from build123d import *

# Parameters (mm, degrees)
SKETCH1_W            = 28
SKETCH1_H            = 22
BOSS_EXTRUDE1_DEPTH  = 32
SKETCH21_W           = 26
SKETCH21_H           = 23
CUT_EXTRUDE10_DEPTH  = 17
SKETCH22_W           = 4
SKETCH22_H           = 8.5
CUT_EXTRUDE11_DEPTH  = 35.885527085
SKETCH23_W           = 10
SKETCH23_H           = 5
CUT_EXTRUDE12_DEPTH  = 5
SKETCH24_W           = 26
SKETCH24_H           = 24
BOSS_EXTRUDE4_DEPTH  = 15
BOSS_EXTRUDE5_DEPTH  = 28
SKETCH26_W           = 28
SKETCH26_H           = 21
SKETCH26_W_2         = 10
SKETCH26_H_2         = 5
BOSS_EXTRUDE6_DEPTH  = 2
BOSS_EXTRUDE7_DEPTH  = 2
FILLET1_R            = 5
FILLET2_R            = 10
SKETCH31_W           = 2
SKETCH31_H           = 26
BOSS_EXTRUDE8_DEPTH  = 0.5
BOSS_EXTRUDE12_DEPTH = 1
SKETCH41_W           = 2
SKETCH41_H           = 4
BOSS_EXTRUDE15_DEPTH = 3.5
SKETCH44_W           = 7
SKETCH44_H           = 6
BOSS_EXTRUDE17_DEPTH = 1
SKETCH30_R           = 1.25
CUT_EXTRUDE13_DEPTH  = 6
BOSS_EXTRUDE9_DEPTH  = 4
SKETCH37_W           = 1
SKETCH37_H           = 27
BOSS_EXTRUDE13_DEPTH = 0.5
SKETCH38_W           = 3
SKETCH38_H           = 2.5
CUT_EXTRUDE15_DEPTH  = 8
CUT_EXTRUDE16_DEPTH  = 6
SKETCH45_W           = 3
SKETCH45_H           = 6
CUT_EXTRUDE18_DEPTH  = 7
BOSS_EXTRUDE18_START = 1
BOSS_EXTRUDE18_DEPTH = 1
SKETCH48_W           = 10
SKETCH48_H           = 5
CUT_EXTRUDE19_DEPTH  = 60.958318856


with BuildPart() as part:
    # Sketch1 → Boss-Extrude1 (new body)
    with BuildSketch(Plane(origin=(0, 0, 0), x_dir=(1, 0, 0), z_dir=(0, 1, 0))):
        Rectangle(SKETCH1_W, SKETCH1_H)
    extrude(amount=BOSS_EXTRUDE1_DEPTH)

    # Sketch21 → Cut-Extrude10 (cut)
    with BuildSketch(Plane.XY.offset(11)):
        with Locations((1, 13.5)):
            Rectangle(SKETCH21_W, SKETCH21_H)
    extrude(amount=-CUT_EXTRUDE10_DEPTH, mode=Mode.SUBTRACT)

    # Sketch22 → Cut-Extrude11 (cut, through all)
    with BuildSketch(Plane(origin=(0, 2, 0), x_dir=(1, 0, 0), z_dir=(0, 1, 0))):
        with Locations((-6, 0)):
            Rectangle(SKETCH22_W, SKETCH22_H)
    extrude(amount=-CUT_EXTRUDE11_DEPTH, mode=Mode.SUBTRACT)

    # Sketch23 → Cut-Extrude12 (cut)
    with BuildSketch(Plane(origin=(0, 0, -11), x_dir=(-1, 0, 0), z_dir=(0, 0, -1))):
        with Locations((0, 16)):
            Rectangle(SKETCH23_W, SKETCH23_H)
    extrude(amount=-CUT_EXTRUDE12_DEPTH, mode=Mode.SUBTRACT)

    # Sketch24 → Boss-Extrude4 (add)
    with BuildSketch(Plane(origin=(14, 0, 0), x_dir=(0, 0, -1), z_dir=(1, 0, 0))):
        with Locations((0, 33)):
            Rectangle(SKETCH24_W, SKETCH24_H)
    extrude(amount=BOSS_EXTRUDE4_DEPTH)

    # Sketch25 → Boss-Extrude5 (add)
    with BuildSketch(Plane.ZY.offset(-14)):
        Polygon((11, 32), (11, 25), (13, 25), (13, 45), (-13, 45), (-13, 21), (-11, 21), (-11, 32), align=None)
    extrude(amount=BOSS_EXTRUDE5_DEPTH)

    # Sketch26 → Boss-Extrude6 (add)
    with BuildSketch(Plane(origin=(0, 0, -11), x_dir=(-1, 0, 0), z_dir=(0, 0, -1))):
        with Locations((0, 10.5)):
            Rectangle(SKETCH26_W, SKETCH26_H)
        with Locations((0, 16)):
            Rectangle(SKETCH26_W_2, SKETCH26_H_2, mode=Mode.SUBTRACT)
    extrude(amount=BOSS_EXTRUDE6_DEPTH)

    # Sketch27 → Boss-Extrude7 (add)
    with BuildSketch(Plane.XY.offset(11)):
        Polygon((14, 0), (-14, 0), (-14, 2), (-14, 25), (-12, 25), (-12, 2), (14, 2), align=None)
    extrude(amount=BOSS_EXTRUDE7_DEPTH)

    # Fillet1
    fillet1_edges = [part.edges().sort_by_distance(p)[0] for p in [
        (-14, 45, 0),
    ]]
    fillet(fillet1_edges, radius=FILLET1_R)

    # Fillet2
    fillet2_edges = [part.edges().sort_by_distance(p)[0] for p in [
        (1, 25, 13),
    ]]
    fillet(fillet2_edges, radius=FILLET2_R)

    # Sketch31 → Boss-Extrude8 (add)
    with BuildSketch(Plane.XZ):
        with Locations((-13, 0)):
            Rectangle(SKETCH31_W, SKETCH31_H)
    extrude(amount=BOSS_EXTRUDE8_DEPTH)

    # Sketch36 → Boss-Extrude12 (add)
    with BuildSketch(Plane.XY.offset(13)):
        Polygon((-12, 2), (-7, 2), (-7, 0), (-12, 0), (-12, -0.5), (-14, -0.5), (-14, 5.5), (-12, 5.5), align=None)
    extrude(amount=BOSS_EXTRUDE12_DEPTH)

    # Sketch41 → Boss-Extrude15 (add)
    with BuildSketch(Plane(origin=(0, 2, 0), x_dir=(1, 0, 0), z_dir=(0, 1, 0))):
        with Locations((-8, -12)):
            Rectangle(SKETCH41_W, SKETCH41_H)
    extrude(amount=BOSS_EXTRUDE15_DEPTH)

    # Sketch44 → Boss-Extrude17 (add)
    with BuildSketch(Plane(origin=(0, 0, -13), x_dir=(-1, 0, 0), z_dir=(0, 0, -1))):
        with Locations((10.5, 2.5)):
            Rectangle(SKETCH44_W, SKETCH44_H)
    extrude(amount=BOSS_EXTRUDE17_DEPTH)

    # Sketch30 → Cut-Extrude13 (cut)
    with BuildSketch(Plane.ZY.offset(14)):
        with Locations((-12, 1)):
            Circle(SKETCH30_R)
        with Locations((12, 1)):
            Circle(SKETCH30_R)
    extrude(amount=-CUT_EXTRUDE13_DEPTH, mode=Mode.SUBTRACT)

    # Sketch32 → Boss-Extrude9 (add)
    with BuildSketch(Plane(origin=(-12, 0, 0), x_dir=(0, 0, -1), z_dir=(1, 0, 0))):
        with BuildLine():
            Line((13, 0), (12.75, 0))
            ThreePointArc((12.75, 0), (12, -0.25), (11.25, 0))
            Line((11.25, 0), (-11.25, 0))
            ThreePointArc((-11.25, 0), (-12, -0.25), (-12.75, 0))
            Line((-12.75, 0), (-14, 0))
            Line((-14, 0), (-14, -0.5))
            Line((-14, -0.5), (13, -0.5))
            Line((13, -0.5), (13, 0))
        make_face()
    extrude(amount=BOSS_EXTRUDE9_DEPTH)

    # Sketch37 → Boss-Extrude13 (add)
    with BuildSketch(Plane.XZ):
        with Locations((-7.5, 0.5)):
            Rectangle(SKETCH37_W, SKETCH37_H)
    extrude(amount=BOSS_EXTRUDE13_DEPTH)

    # Sketch38 → Cut-Extrude15 (cut)
    with BuildSketch(Plane.XY.offset(14)):
        with Locations((-10.5, 0.75)):
            Rectangle(SKETCH38_W, SKETCH38_H)
    extrude(amount=-CUT_EXTRUDE15_DEPTH, mode=Mode.SUBTRACT)

    # Sketch39 → Cut-Extrude16 (cut)
    with BuildSketch(Plane.ZY.offset(-14)):
        with BuildLine():
            Line((13, 21), (13, 35))
            ThreePointArc((13, 35), (10.071067812, 27.928932188), (3, 25))
            Line((3, 25), (-6, 25))
            Line((-6, 25), (-6, 21))
            Line((-6, 21), (13, 21))
        make_face()
    extrude(amount=-CUT_EXTRUDE16_DEPTH, mode=Mode.SUBTRACT)

    # Sketch45 → Cut-Extrude18 (cut)
    with BuildSketch(Plane(origin=(0, 0, -14), x_dir=(-1, 0, 0), z_dir=(0, 0, -1))):
        with Locations((10.5, 2.5)):
            Rectangle(SKETCH45_W, SKETCH45_H)
    extrude(amount=-CUT_EXTRUDE18_DEPTH, mode=Mode.SUBTRACT)

    # Sketch46 → Boss-Extrude18 (add)
    with BuildSketch(Plane(origin=(0, 0, -13), x_dir=(-1, 0, 0), z_dir=(0, 0, -1)).offset(BOSS_EXTRUDE18_START)):
        with BuildLine():
            Line((7, 0), (7, 5.5))
            Line((7, 5.5), (9, 5.5))
            Line((9, 5.5), (12, 5.5))
            Line((12, 5.5), (14, 5.5))
            Line((14, 5.5), (14, 40))
            ThreePointArc((14, 40), (12.535533906, 43.535533906), (9, 45))
            Line((9, 45), (-29, 45))
            Line((-29, 45), (-29, 21))
            Line((-29, 21), (-14, 21))
            Line((-14, 21), (-14, 0))
            Line((-14, 0), (7, 0))
        make_face()
    extrude(amount=-BOSS_EXTRUDE18_DEPTH)

    # Sketch48 → Cut-Extrude19 (cut, through all)
    with BuildSketch(Plane.XY.offset(-13)):
        with Locations((0, 16)):
            Rectangle(SKETCH48_W, SKETCH48_H)
    extrude(amount=-CUT_EXTRUDE19_DEPTH, mode=Mode.SUBTRACT)


solid = part.part
Source: CAD feature listing. Evaluate the final solid. Frame: model axes, mm. A direction names the side the tool comes from. Give positions to 0.01 mm unless a question says otherwise; leave off trailing zeros. Order: outer loops, then holes, each group sorted by start corner. A loop starts at its lowest first (then second) coordinate and runs counter-clockwise, first axis right, second up. Notation, with made-up numbers: (53.5, 50.5) -> (102.5, 50.5) arc R22 cw to (102.5, 79.5) -> close; hole circle Ø7 at (-1, 16.25). An arc over 180 degrees is marked (long way). Write item = value, one per line.
Q1. Material intervals for line 1 (Z direction, x = -8.5, y = 1); line 2 (X direction, y = 22, z = 1.25); line 3 (Y direction, x = -8.65, z = -12), sorted ascending. Write a range as from..to.
Data:
line_1 = -14..-13.25, -10.75..10.75, 13.25..14
line_2 = -14..-12, 20..29
line_3 = -0.5..-0.25, 2.25..45
Q2. Pull-direction query (X, two-part tool) for faces 1 (the face through (-8, 3, 14)), 2 (the face through (-8, 1, 12)), 3 (the face through (-6, 1, 4.25)), 4 (the face through (-4, 1, 0)); classes: released by +X, released by -X, zero draft, split by the parting line, or undercut.
Data:
face_1 = zero draft
face_2 = released by -X
face_3 = undercut
face_4 = undercut
Q3. Cut plane C-C, the plane y = 15. Output: boundary loops of the cut face in (x, z).
Data:
outline = (-14, -14) -> (-5, -14) -> (-5, -6) -> (-12, -6) -> (-12, 13) -> (-14, 13) -> close; (5, -14) -> (14, -14) -> (14, -6) -> (5, -6) -> close
Q4. Pin query (flat end, axial travel): pin 1 (1.5 mm diameter, centred on x = -0.5, z = -5.5, fed in from -Y); pin 2 (12 mm diameter, centred on x = -0.5, y = 33.5, fed in from +Z); pin 3 (0.8 mm diameter, centred on y = 1.5, z = 11.5, fed in from -X). Return the tip coordinate at first contact, or that it passes through.
Data:
pin_1 = 0
pin_2 = 13
pin_3 = -8
Q5. Cut plane B-B, the plane x = 2. Output: boundary loops of the cut face in (y, z).
Data:
outline = (0, -14) -> (13.5, -14) -> (13.5, -6) -> (2, -6) -> (2, 13) -> (0, 13) -> close; (18.5, -14) -> (45, -14) -> (45, 13) -> (35, 13) arc R10 ccw to (25, 3) -> (25, -6) -> (18.5, -6) -> close
Q6. Cut plane A-A, the plane z = -12. Output: boundary loops of the cut face in (x, y).
Data:
outline = (-14, -0.5) -> (-12, -0.5) -> (-12, -0.25) -> (-14, -0.25) -> close; (-14, 2.25) -> (-12, 2.25) -> (-12, 5.5) -> (-9, 5.5) -> (-9, 2.25) -> (-8, 2.25) -> (-8, -0.25) -> (-9, -0.25) -> (-9, -0.5) -> (-7, -0.5) -> (-7, 0) -> (14, 0) -> (14, 21) -> (29, 21) -> (29, 45) -> (-9, 45) arc R5 ccw to (-14, 40) -> close; hole (-5, 13.5) -> (5, 13.5) -> (5, 18.5) -> (-5, 18.5) -> close
Q7. Cut plane D-D, the plane z = -2.75. Output: boundary loops of the cut face in (x, y).
Data:
outline = (-14, -0.5) -> (-7, -0.5) -> (-7, 0) -> (-8, 0) -> (-8, 2) -> (-12, 2) -> (-12, 25) -> (20, 25) -> (20, 21) -> (29, 21) -> (29, 45) -> (-9, 45) arc R5 ccw to (-14, 40) -> close; (-4, 0) -> (14, 0) -> (14, 2) -> (-4, 2) -> close
Q8. Set-up query: faces 5 (the face through (-11, 1, 6)), 6 (the face through (-5, 16, -10)), 7 (the face through (11, 36, 13)). Return all of +Z, -Z, +X, -X, +Y, -Y with unobstructed straight access to the full face (end or side cutting, diameter ignored); none if empty.
Data:
face_5 = +Z, -Y
face_6 = +Z, -Z
face_7 = +Z, +X, -X, +Y
